Job drawing, mm, ordinate dimensions from the low corner. One solid piece. A direction names the side the tool comes from. Give positions to 0.01 mm unless a question says otherwise; leave off trailing zeros. Order: outer loops, then holes, each group sorted by start corner. A loop starts at its lowest first (then second) coordinate and runs counter-clockwise, first axis right, second up. Notation, with made-up numbers: (-1, 8.5) - (38, 8.5) arc R28 cw to (38, 41.5) - close; hole circle Ø3 at (-10, -29.5). An arc over 180 degrees is marked (long way). One line per item, written item: value.
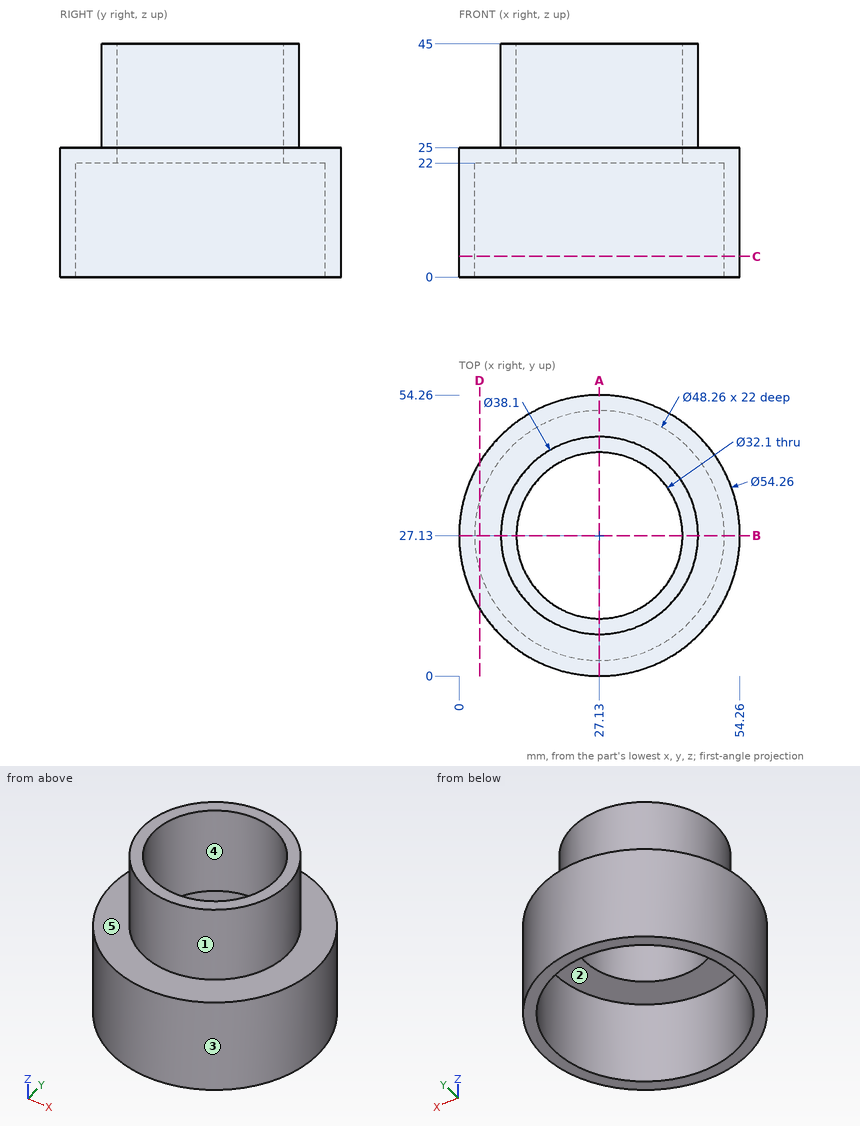
1) Two-plate mould, pull along Y, no slides. Class the marked faces 3, 4 and 5: pulls with the +Y half, pulls with the -Y half, needs draft (parallel to the pull), parting line crosses it, or undercut.
Answer:
face 3: parting line crosses it
face 4: undercut
face 5: needs draft
2) Slice it at D-D on x = 4. Write the cut outline in (y, z).
Answer:
outline: (12.95, 0) - (20.26, 0) - (20.26, 22) - (34, 22) - (34, 0) - (41.31, 0) - (41.31, 25) - (12.95, 25) - close
3) Drop flat-ended pins along their axis: P1, Ø2, axis at x = 42.5, z = 11, coming from the -Y side; P2, Ø6, axis at x = 35, y = 37, coming from the -Z side; P3, Ø4, axis at x = 8.5, y = 9.5, coming from the +Z side; P4, Ø14.5, axis at x = 36, y = 16, coming from the -Z side. Give the stop position or say it passes through.
Answer:
P1: stops at y = 4.12
P2: passes through
P3: stops at z = 25
P4: stops at z = 22
4) Slice it at C-C on z = 4. Write the cut outline in (x, y), then the cut area to 3 significant figures.
Answer:
outline: circle Ø54.26 at (27.13, 27.13); hole circle Ø48.26 at (27.13, 27.13)
area: 483 mm2
5) Which spindle directions (+Z, -Z, +X, -X, +Y, -Y) get a long thin tool onto all of the face, cutting with end or side? Do the marked faces 1 and 2. Say none if no direction does.
Answer:
face 1: +Z
face 2: -Z
6) Slice it at A-A on x = 27.13. Write the cut outline in (y, z).
Answer:
outline: (0, 0) - (3, 0) - (3, 22) - (11.08, 22) - (11.08, 45) - (8.08, 45) - (8.08, 25) - (0, 25) - close; (43.18, 22) - (51.26, 22) - (51.26, 0) - (54.26, 0) - (54.26, 25) - (46.18, 25) - (46.18, 45) - (43.18, 45) - close
7) Wall check: line 1 along X through (y, z) = (26.5, 18); line 2 along Y through (x, z) = (27, 27); line 3 along Y through (x, z) = (27, 4). Give the ranges that are in metal, low to high. Write a range as [from, to].
Answer:
line 1: x = [0.01, 3.01], [51.25, 54.25]
line 2: y = [8.08, 11.08], [43.18, 46.18]
line 3: y = [0, 3], [51.26, 54.26]
